Autodesk Inventor part; units mm, degrees
ref_plane "YZ Plane" through (0, 0, 0) normal (1, 0, 0) x (0, 1, 0)
ref_plane "XZ Plane" through (0, 0, 0) normal (0, 1, 0) x (-1, 0, 0)
ref_plane "XY Plane" through (0, 0, 0) normal (0, 0, 1) x (1, 0, 0)
ref_plane "Work Plane1" through (-136.8843, -40.4621, -113.009) normal (0, 0, 1) x (1, 0, 0)
sketch "Sketch1" plane through (-136.8843, -40.4621, -113.009) normal (0, 0, 1) x (1, 0, 0)
  line L0 (-25, -40) -> (25, -40)
  line L1 (25, -40) -> (25, 40)
  line L2 (25, 40) -> (-25, 40)
  line L3 (-25, 40) -> (-25, -40)
  line L4 (-25, -40) -> (25, 40) construction
  line L5 (25, -40) -> (-25, 40) construction
  point P0 (136.8843, 40.4621)
  point P1 (0, 0)
  dimension "d0" = 50
  dimension "d1" = 80
extrude "Extrusion1" add sketch "Sketch1" along normal blind 15
fillet "Fillet1" radius 8 4 edges at (-136.8843, -80.4621, -98.009) (-111.8843, -40.4621, -98.009) (-136.8843, -0.4621, -98.009) (-161.8843, -40.4621, -98.009)
properties part number "rubber padding"
Work out the finished part from the listing and answer in its coordinate system (mm). Round coordinates to 2 decimals unless told otherwise and drop trailing zeros. Loops run counter-clockwise (first coordinate to the right, second up) from the corner with the lowest first, then second, coordinate; pieces in that order, holes last. Notation, with made-up numbers: (1, 33) -> (58, 33) arc R11 cw to (58, 37) -> close; hole circle Ø1 at (28.25, 58). An arc over 180 degrees is marked (long way). Write each question's results on one line, items separated by ' | '. Start each with the question number.
1. Section C-C (z = -102.25) is taken. Determine the outline of the cut face in (x, y), plus the area to 3 significant figures.
2. Given pin 1 Ø5 at (x, z) = (-130.5, -101.5) entering from -Y; pin 2 Ø2 at (x, z) = (-149.5, -103.5) entering from +Y; pin 3 Ø4 at (y, z) = (-44.5, -103) entering from +X, each flat-ended and moving along its own axis, determine where each tip first touches the part or whether it passes through.
3. Find the intervals of material crossed by probe 1 along Z at (x, y) = (-154, -60); probe 2 along X at (y, z) = (-36, -104.75); probe 3 along X at (y, z) = (-9.5, -99), in increasing order. Write a range as from..to.
4. Section B-B (x = -144) is taken. Determine the outline of the cut face in (y, z).
5. Section A-A (y = -64.5) is taken. Determine the outline of the cut face in (x, z).
Evaluation:
1) outline: (-160.95, -79.52) -> (-112.82, -79.52) -> (-112.82, -1.4) -> (-160.95, -1.4) -> close | area: 3,760 mm2
2) pin 1: stops at y = -80.21 | pin 2: stops at y = -0.61 | pin 3: stops at x = -111.95
3) probe 1: z = -113.01..-98.01 | probe 2: x = -161.78..-111.98 | probe 3: x = -157.74..-116.03
4) outline: (-80.46, -113.01) -> (-0.46, -113.01) -> (-0.46, -106.01) arc R8 ccw to (-8.46, -98.01) -> (-72.46, -98.01) arc R8 ccw to (-80.46, -106.01) -> close
5) outline: (-161.88, -113.01) -> (-111.88, -113.01) -> (-111.88, -106.01) arc R8 ccw to (-119.88, -98.01) -> (-153.88, -98.01) arc R8 ccw to (-161.88, -106.01) -> close
